Autodesk Inventor part; units mm, degrees
ref_plane "YZ Plane" through (0, 0, 0) normal (1, 0, 0) x (0, 1, 0)
ref_plane "XZ Plane" through (0, 0, 0) normal (0, 1, 0) x (-1, 0, 0)
ref_plane "XY Plane" through (0, 0, 0) normal (0, 0, 1) x (1, 0, 0)
sketch "Skizze1" plane through (0, 0, 0) normal (0, 0, 1) x (1, 0, 0)
  line L0 (-17.75, 16.5) -> (17.75, 16.5)
  line L1 (17.75, 16.5) -> (17.75, -16.5)
  line L2 (17.75, -16.5) -> (-17.75, -16.5)
  line L3 (-17.75, -16.5) -> (-17.75, 16.5)
  line L4 (-17.75, 16.5) -> (17.75, -16.5) construction
  line L5 (17.75, 16.5) -> (-17.75, -16.5) construction
  point P0 (0, 0)
  dimension "d0" = 33
  dimension "d1" = 35.5
extrude "Extrusion1" add sketch "Skizze1" along normal blind 1
sketch "Skizze2" plane through (0, 0, 1) normal (0, 0, 1) x (1, 0, 0)
  line L0 (-17.75, 16.5) -> (-17.75, -16.5)
  line L1 (17.75, -16.5) -> (17.75, 16.5)
  line L2 (-17.75, 11) -> (17.75, 11)
  line L3 (17.75, 11) -> (17.75, -12)
  line L4 (17.75, -12) -> (-17.75, -12)
  line L5 (-17.75, -12) -> (-17.75, 11)
  line L6 (17.75, 16.5) -> (-17.75, 16.5)
  line L7 (-7, -14.5) -> (7, -14.5)
  line L8 (7, -14.5) -> (7, -12)
  line L9 (7, -12) -> (-7, -12)
  line L10 (-7, -12) -> (-7, -14.5)
  line L11 (-7, -14.5) -> (7, -12) construction
  line L12 (7, -14.5) -> (-7, -12) construction
  line L13 (-17.75, -16.5) -> (17.75, -16.5)
  point P0 (0, 0)
  point P1 (0, -13.25)
  point P2 (0, -13.25)
  point P3 (17.75, 11)
  point P4 (-17.75, -12)
  point P5 (-7, -12)
  dimension "d4" = 23
  dimension "d5" = 5.5
  dimension "d6" = 14
  dimension "d7" = 2
extrude "Extrusion2" add sketch "Skizze2" along normal blind 2 contours L2 L1 L4 L0 | L4 L8 L7 L10
sketch "Skizze3" plane through (0, 0, 0) normal (0, 0, -1) x (-1, 0, 0)
  line L0 (-17.75, 16.5) -> (17.75, 16.5)
  line L1 (-5.5, 14) -> (5.5, 14)
  line L2 (5.5, 14) -> (5.5, 16.5)
  line L3 (5.5, 16.5) -> (-5.5, 16.5)
  line L4 (-5.5, 16.5) -> (-5.5, 14)
  line L5 (-5.5, 14) -> (5.5, 16.5) construction
  line L6 (5.5, 14) -> (-5.5, 16.5) construction
  point P0 (0, 0)
  point P1 (0, 15.25)
  point P2 (0, 15.25)
  dimension "d10" = 11
  dimension "d11" = 2.5
extrude "Extrusion3" add sketch "Skizze3" along normal blind 15
sketch "Skizze4" plane through (0, 0, 1) normal (0, 0, 1) x (1, 0, 0)
  line L0 (-15, 14) -> (15, 14)
  line L1 (15, 14) -> (15, -14)
  line L2 (15, -14) -> (-15, -14)
  line L3 (-15, -14) -> (-15, 14)
  line L4 (-15, 14) -> (15, -14) construction
  line L5 (15, 14) -> (-15, -14) construction
  point P0 (0, 0)
  dimension "d14" = 28
  dimension "d15" = 30
hole "Bohrung1" at (-15, 14, 1) at (15, 14, 1) at (15, -14, 1) at (-15, -14, 1) direction (0, 0, -1) diameter 2.9 end through all
properties part number "display" material "Glas"
Geometry: final body of the model. Coordinates: model frame, mm. A direction names the side the tool comes from. Coordinates: 2 decimals unless noted, no trailing zeros. Order: outer loops, then holes, each group sorted by start corner. A loop starts at its lowest first (then second) coordinate and runs counter-clockwise, first axis right, second up. Notation, with made-up numbers: (39, -24) - (49, -24) arc R33 cw to (49, 6) - close; hole circle Ø7 at (89, 52.5). An arc over 180 degrees is marked (long way). Write each question's results on one line, items separated by ' | '.
(1) Section query B-B, the plane y = -14. Return the cut outline in (x, z), plus the area to 3 significant figures.
Values found:
outline: (-17.75, 0) - (-16.45, 0) - (-16.45, 1) - (-17.75, 1) - close; (-13.55, 0) - (13.55, 0) - (13.55, 1) - (7, 1) - (7, 3) - (-7, 3) - (-7, 1) - (-13.55, 1) - close; (16.45, 0) - (17.75, 0) - (17.75, 1) - (16.45, 1) - close | area: 57.7 mm²
(2) Section query A-A, the plane x = -2. Return the cut outline in (y, z).
Values found:
outline: (-16.5, 0) - (14, 0) - (14, -15) - (16.5, -15) - (16.5, 1) - (11, 1) - (11, 3) - (-14.5, 3) - (-14.5, 1) - (-16.5, 1) - close
(3) Line query: line 1 (Y direction, x = -15, z = 0.7); line 2 (X direction, y = -14, z = 0.6); line 3 (Z direction, x = 4, y = -9.5). Output: solid intervals per line, ascending. Write a range as [from, to].
Values found:
line 1: y = [-16.5, -15.45], [-12.55, 12.55], [15.45, 16.5] | line 2: x = [-17.75, -16.45], [-13.55, 13.55], [16.45, 17.75] | line 3: z = [0, 3]
(4) Section query D-D, the plane x = 15. Return the cut outline in (y, z), plus the area to 3 significant figures.
Values found:
outline: (-16.5, 0) - (-15.45, 0) - (-15.45, 1) - (-16.5, 1) - close; (-12.55, 0) - (12.55, 0) - (12.55, 1) - (11, 1) - (11, 3) - (-12, 3) - (-12, 1) - (-12.55, 1) - close; (15.45, 0) - (16.5, 0) - (16.5, 1) - (15.45, 1) - close | area: 73.2 mm²
(5) Section query C-C, the plane z = 0.5. Return the cut outline in (x, y).
Values found:
outline: (-17.75, -16.5) - (17.75, -16.5) - (17.75, 16.5) - (-17.75, 16.5) - close; hole circle Ø2.9 at (-15, -14); hole circle Ø2.9 at (-15, 14); hole circle Ø2.9 at (15, -14); hole circle Ø2.9 at (15, 14)
(6) First-contact query: pin 1 Ø1.5 at (x, z) = (5.5, -3.5) entering from -Y; pin 2 Ø1.6 at (y, z) = (-13, 2) entering from -X; pin 3 Ø1.7 at (x, y) = (-15, 14) entering from -Z; pin 4 Ø8 at (x, z) = (8, -2) entering from +Y. Flat tips, straight axial feed; report the tip coordinate or a pass-through.
Values found:
pin 1: stops at y = 14 | pin 2: stops at x = -7 | pin 3: passes through | pin 4: stops at y = 16.5
(7) Set-up query: faces 1 (the face through (12, -12, 2)), 2 (the face through (-7, -13, 2)), 3 (the face through (5.5, 15, -7)). Return all of +Z, -Z, +X, -X, +Y, -Y with unobstructed straight access to the full face (end or side cutting, diameter ignored); none if empty.
Values found:
face 1: +Z, +X, -Y | face 2: +Z, -X, -Y | face 3: -Z, +X, +Y, -Y
(8) Mould query, pull axis Y, two halves, no side actions, for faces 4 (the face through (0, 11, 2)), 5 (the face through (0, 15, -15)), 6 (the face through (-12, -12, 2)), 7 (the face through (-15.44, 12.62, 0.49)). Classes: +Y half, -Y half, draft (parallel to the pull), parting line (faces both ways), or undercut.
Values found:
face 4: +Y half | face 5: draft | face 6: -Y half | face 7: undercut
